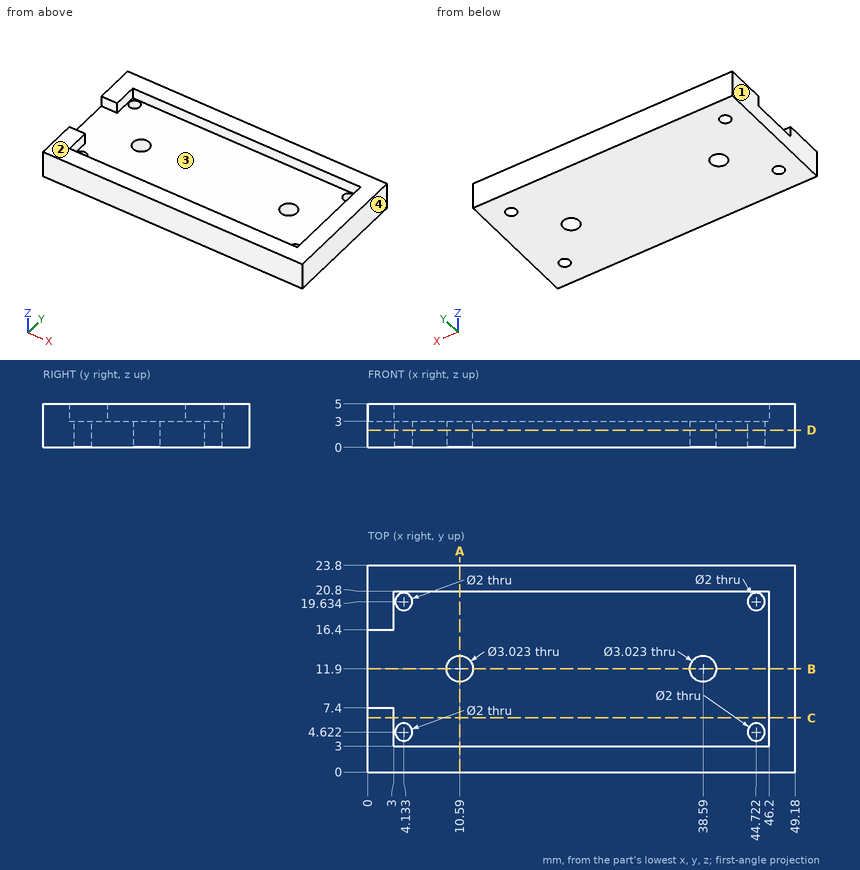
Here's the drawing with two shaded views (mm, measured from the low corner). I have some questions. Coordinates: 2 decimals unless noted, no trailing zeros. Loops run counter-clockwise (first coordinate to the right, second up) from the corner with the lowest first, then second, coordinate; pieces in that order, holes last. Notation, with made-up numbers: (53.25, -4) -> (60.25, -4) arc R26 ccw to (60.25, 20) -> close; hole circle Ø3 at (-4, -3). An arc over 180 degrees is marked (long way). Answer as a JSON object with one key per item and string values.
1) Imagine slicing it at C-C (y = 6.25). Please give me the cut outline in (x, z).
Results:
{"outline": "(0, 0) -> (49.18, 0) -> (49.18, 5) -> (46.2, 5) -> (46.2, 3) -> (3, 3) -> (3, 5) -> (0, 5) -> close"}
2) For P1, Ø1.2, axis at x = 44.72, y = 19.63, coming from the +Z side; P2, Ø1, axis at y = 14.5, z = 4.5, coming from the -X side; P3, Ø4, axis at x = 38.59, y = 11.9, coming from the +Z side, each with a flat end and sliding along its axis, tell me the tip position at first contact or that it passes through.
Results:
{"P1": "passes through", "P2": "stops at x = 46.2", "P3": "stops at z = 3"}
3) Thinking about a two-plate mould opening in X: for the marked faces 1, 2, 3 and 4, which applies, pulls with the +X half, pulls with the -X half, needs draft (parallel to the pull), parting line crosses it, or undercut?
Results:
{"face 1": "pulls with the -X half", "face 2": "needs draft", "face 3": "undercut", "face 4": "pulls with the +X half"}
4) If I drill on line 1 (X direction, y = 3.75, z = 3.75); line 2 (X direction, y = 11.9, z = 0.85); line 3 (Y direction, x = 38.59, z = 1.95), over which ranges is the centre line in solid material (lowest first)?
Results:
{"line 1": "x = 0 to 3, 46.2 to 49.18", "line 2": "x = 0 to 9.08, 12.1 to 37.08, 40.1 to 49.18", "line 3": "y = 0 to 10.39, 13.41 to 23.8"}
5) Imagine slicing it at D-D (z = 2). Please give me the cut outline in (x, y) (1 decimal), then the cut area to 3 significant figures.
Results:
{"outline": "(0, 0) -> (49.2, 0) -> (49.2, 23.8) -> (0, 23.8) -> close; hole circle Ø2 at (4.1, 4.6); hole circle Ø2 at (4.1, 19.6); hole circle Ø3 at (10.6, 11.9); hole circle Ø3 at (38.6, 11.9); hole circle Ø2 at (44.7, 4.6); hole circle Ø2 at (44.7, 19.6)", "area": "1,140 mm^2"}
6) Imagine slicing it at A-A (x = 10.59). Please give me the cut outline in (y, z).
Results:
{"outline": "(0, 0) -> (10.39, 0) -> (10.39, 3) -> (3, 3) -> (3, 5) -> (0, 5) -> close; (13.41, 0) -> (23.8, 0) -> (23.8, 5) -> (20.8, 5) -> (20.8, 3) -> (13.41, 3) -> close"}
7) Imagine slicing it at B-B (y = 11.9). Please give me the cut outline in (x, z).
Results:
{"outline": "(0, 0) -> (9.08, 0) -> (9.08, 3) -> (0, 3) -> close; (12.1, 0) -> (37.08, 0) -> (37.08, 3) -> (12.1, 3) -> close; (40.1, 0) -> (49.18, 0) -> (49.18, 5) -> (46.2, 5) -> (46.2, 3) -> (40.1, 3) -> close"}
